```python
from build123d import *

# Parameters (mm, degrees)
BOSS_EXTRUDE1_DEPTH = 3.175
FILLET1_R           = 38.1
SKETCH2_W           = 42.672654426
SKETCH2_H           = 6.35
CUT_EXTRUDE1_DEPTH  = 3.175
BOSS_EXTRUDE2_DEPTH = 3.175


with BuildPart() as part:
    # Sketch1 → Boss-Extrude1 (new body)
    with BuildSketch(Plane.XY):
        with BuildLine():
            Line((-221.658355151, 4.726030951), (-123.220415709, 91.814619456))
            ThreePointArc((-123.220415709, 91.814619456), (-126.780447272, 102.154073831), (-121.98667143, 111.982494593))
            Line((-121.98667143, 111.982494593), (-137.765113811, 129.81717744))
            Line((-137.765113811, 129.81717744), (-257.60467267, 23.794458078))
            Line((-257.60467267, 23.794458078), (-241.826230288, 5.95977523))
            ThreePointArc((-241.826230288, 5.95977523), (-231.486775913, 9.519806794), (-221.658355151, 4.726030951))
        make_face()
        with BuildLine():
            Line((-207.113657049, -33.276527034), (-87.274098191, 72.746192329))
            Line((-87.274098191, 72.746192329), (-103.052540572, 90.580875176))
            ThreePointArc((-103.052540572, 90.580875176), (-113.391994947, 87.020843613), (-123.220415709, 91.814619456))
            Line((-123.220415709, 91.814619456), (-221.658355151, 4.726030951))
            ThreePointArc((-221.658355151, 4.726030951), (-218.998392521, 0.320824743), (-218.071664859, -4.741034478))
            ThreePointArc((-218.071664859, -4.741034478), (-219.332397157, -10.60925222), (-222.892099431, -15.441844187))
            Line((-222.892099431, -15.441844187), (-207.113657049, -33.276527034))
        make_face()
        with BuildLine():
            Line((-226.137318753, -50.106865574), (-207.113657049, -33.276527034))
            Line((-207.113657049, -33.276527034), (-222.892099431, -15.441844187))
            ThreePointArc((-222.892099431, -15.441844187), (-233.231553806, -19.00187575), (-243.059974568, -14.208099907))
            Line((-243.059974568, -14.208099907), (-251.382826563, -21.571373018))
            Line((-251.382826563, -21.571373018), (-226.137318753, -50.106865574))
        make_face()
        with BuildLine():
            Line((-251.382826563, -21.571373018), (-243.059974568, -14.208099907))
            ThreePointArc((-243.059974568, -14.208099907), (-246.620006131, -3.868645532), (-241.826230288, 5.95977523))
            Line((-241.826230288, 5.95977523), (-257.60467267, 23.794458078))
            Line((-257.60467267, 23.794458078), (-276.628334373, 6.964119538))
            Line((-276.628334373, 6.964119538), (-251.382826563, -21.571373018))
        make_face()
        with BuildLine():
            Line((-101.818796292, 110.748750313), (-93.495944297, 118.112023425))
            Line((-93.495944297, 118.112023425), (-118.741452107, 146.647515981))
            Line((-118.741452107, 146.647515981), (-137.765113811, 129.81717744))
            Line((-137.765113811, 129.81717744), (-121.98667143, 111.982494593))
            ThreePointArc((-121.98667143, 111.982494593), (-111.647217054, 115.542526156), (-101.818796292, 110.748750313))
        make_face()
        with BuildLine():
            Line((-103.052540572, 90.580875176), (-87.274098191, 72.746192329))
            Line((-87.274098191, 72.746192329), (-68.250436487, 89.576530869))
            Line((-68.250436487, 89.576530869), (-93.495944297, 118.112023425))
            Line((-93.495944297, 118.112023425), (-101.818796292, 110.748750313))
            ThreePointArc((-101.818796292, 110.748750313), (-99.158833662, 106.343544105), (-98.232106001, 101.281684885))
            ThreePointArc((-98.232106001, 101.281684885), (-99.492838298, 95.413467143), (-103.052540572, 90.580875176))
        make_face()
    extrude(amount=BOSS_EXTRUDE1_DEPTH)

    # Fillet1
    fillet1_edges = [part.edges().sort_by_distance(p)[0] for p in [
        (-276.628334373, 6.964119538, 1.5875),
        (-226.137318753, -50.106865574, 1.5875),
        (-68.250436487, 89.576530869, 1.5875),
        (-118.741452107, 146.647515981, 1.5875),
    ]]
    fillet(fillet1_edges, radius=FILLET1_R - 0.0001)  # a hair under: the kernel refuses the full size

    # Sketch2 → Cut-Extrude1 (cut)
    with BuildSketch(Plane.XY.offset(3.175)):
        with Locations((-222.571574213, -31.250865208)):
            Rectangle(SKETCH2_W, SKETCH2_H)
    extrude(amount=-CUT_EXTRUDE1_DEPTH, mode=Mode.SUBTRACT)


with BuildPart() as cut_extrude1_kept_piece:
    # of the separate pieces the step leaves, the one the design keeps (cut_extrude1_pieces_kept)
    add(part.part.solids().sort_by_distance((-251.382760302, -21.571447914, 0))[0])

    # Sketch3 → Boss-Extrude2 (add)
    with BuildSketch(Plane.XY.offset(3.175)):
        with BuildLine():
            Line((-84.386706387, -28.075865208), (-84.386706387, 86.994184885))
            ThreePointArc((-84.386706387, 86.994184885), (-88.606891327, 74.579641731), (-96.785929043, 64.331023059))
            Line((-96.785929043, 64.331023059), (-197.601826197, -24.861357764))
            ThreePointArc((-197.601826197, -24.861357764), (-199.63857671, -26.541152476), (-201.786766589, -28.075865208))
            Line((-201.786766589, -28.075865208), (-84.386706387, -28.075865208))
        make_face()
    extrude(amount=-BOSS_EXTRUDE2_DEPTH)


solid = cut_extrude1_kept_piece.part
```
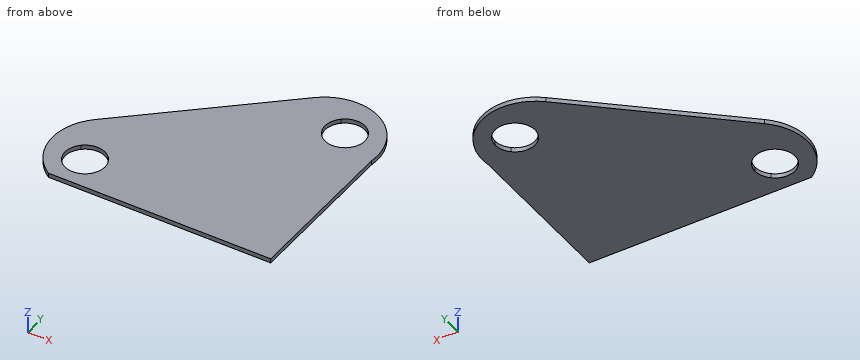
CAD build for the part. Positions are in the model's coordinates, mm. Round coordinates to 2 decimals unless told otherwise and drop trailing zeros. Order: outer loops, then holes, each group sorted by start corner. A loop starts at its lowest first (then second) coordinate and runs counter-clockwise, first axis right, second up. Notation, with made-up numbers: (48.5, 79) -> (58.5, 79) arc R35 ccw to (58.5, 117) -> close; hole circle Ø1 at (-18, 1). An arc over 180 degrees is marked (long way). Write item = value, one per line.
(1) Cut at C-C (y = 47). Write the cut outline in (x, z) (3 decimals).
Answers follow:
outline = (-231.375, 0) -> (-84.387, 0) -> (-84.387, 3.175) -> (-231.375, 3.175) -> close
(2) Cut at A-A (x = -232.5). Write the cut outline in (y, z) (3 decimals), plus the area to 3 significant figures.
Answers follow:
outline = (-28.076, 0) -> (-19.028, 0) -> (-19.028, 3.175) -> (-28.076, 3.175) -> close; (9.546, 0) -> (46.005, 0) -> (46.005, 3.175) -> (9.546, 3.175) -> close
area = 144 mm²
(3) Cut at B-B (z = 2.4). State how many separate pieces and enclosed holes the cut face has, plus the area to 3 significant figures.
Answers follow:
separate_pieces = 1
enclosed_holes = 2
area = 19,400 mm²
(4) Cut at D-D (x = -177). Write the cut outline in (y, z) (3 decimals).
Answers follow:
outline = (-28.076, 0) -> (95.106, 0) -> (95.106, 3.175) -> (-28.076, 3.175) -> close
(5) Flat gauge pins, fed straight in: P1, Ø1.6, axis at y = 1.5, z = 1, coming from the +X side; P2, Ø1, axis at y = 108.5, z = 0.5, coming from the +X side. Where does each tip first touch, or does it go through?
Answers follow:
P1 = -84.39
P2 = -87.07
(6) Drill centre lines: L1, parallel to Y at x = -119, z = 2.9 (3 decimals); L2, parallel to Y at x = -114, z = 1.4; L3, parallel to X at y = 33.5, z = 2.95. Where is each one in solid material? Low to high.
Answers follow:
L1 = -28.076 to 88.548, 114.015 to 130.846
L2 = -28.08 to 87.07, 115.49 to 130.11
L3 = -246.63 to -84.39
